```python
from build123d import *

# Parameters (mm, degrees)
SKETCH1_W           = 14.3764
SKETCH1_H           = 14.478
SKETCH1_R           = 0.889
BOSS_EXTRUDE1_DEPTH = 1.8415
SKETCH2_R           = 0.92075
BOSS_EXTRUDE2_DEPTH = 1.27
SKETCH2_4_R         = 0.92075
BOSS_EXTRUDE3_DEPTH = 3.175
FILLET1_R           = 0.762
FILLET2_R           = 0.254


with BuildPart() as part:
    # Sketch1 → Boss-Extrude1 (new body)
    with BuildSketch(Plane(origin=(0, 0, 0), x_dir=(1, 0, 0), z_dir=(0, 1, 0))):
        Rectangle(SKETCH1_W, SKETCH1_H)
        with Locations((-2.6162, 5.1435)):
            Circle(SKETCH1_R, mode=Mode.SUBTRACT)
        with Locations((-2.6162, -5.1435)):
            Circle(SKETCH1_R, mode=Mode.SUBTRACT)
    extrude(amount=BOSS_EXTRUDE1_DEPTH)

    # Sketch2 → Boss-Extrude2 (add, symmetric)
    with BuildSketch(Plane.XY):
        with BuildLine():
            Line((0.848172569, 7.926885609), (-4.6482, 1.8415))
            Line((-4.6482, 1.8415), (5.93687295, 1.8415))
            Line((5.93687295, 1.8415), (5.93687295, 5.969))
            ThreePointArc((5.93687295, 5.969), (4.064774324, 8.695178077), (0.848172569, 7.926885609))
        make_face()
        with Locations((3.01587295, 5.969)):
            Circle(SKETCH2_R, mode=Mode.SUBTRACT)
    extrude(amount=BOSS_EXTRUDE2_DEPTH, both=True)

    # Sketch2<4> → Boss-Extrude3 (add, symmetric)
    with BuildSketch(Plane.XY):
        with Locations((3.01587295, 5.969)):
            Circle(SKETCH2_4_R)
    extrude(amount=BOSS_EXTRUDE3_DEPTH, both=True)

    # Fillet1
    fillet1_edges = [part.edges().sort_by_distance(p)[0] for p in [
        (7.1882, 1.8415, 0),
        (0, 1.8415, -7.239),
        (-4.6482, 1.8415, 0),
        (-7.1882, 1.8415, 0),
        (-7.1882, 0.92075, -7.239),
        (7.1882, 0.92075, -7.239),
        (7.1882, 0.92075, 7.239),
        (-7.1882, 0.92075, 7.239),
        (0, 1.8415, 7.239),
    ]]
    fillet(fillet1_edges, radius=FILLET1_R)

    # Fillet2
    fillet2_edges = [part.edges().sort_by_distance(p)[0] for p in [
        (2.09512295, 5.969, -3.175),
        (2.09512295, 5.969, 3.175),
    ]]
    fillet(fillet2_edges, radius=FILLET2_R)


solid = part.part
```
Can you work these out from the model? Positions are in its coordinate system, mm. A direction names the side the tool comes from. Coordinates: 2 decimals unless noted, no trailing zeros. Loops run counter-clockwise (first coordinate to the right, second up) from the corner with the lowest first, then second, coordinate; pieces in that order, holes last. Notation, with made-up numbers: (-2.75, 11.5) - (42.25, 11.5) arc R19 ccw to (42.25, 31.5) - close; hole circle Ø1 at (-17, 30.25). An arc over 180 degrees is marked (long way). Answer as CSV lines item,"result". Start each with the question number.
1) Thinking about a two-plate mould opening in Z: for faces 1 (the cylindrical face through (2.82, 5.07, 2.11)), 2 (the flat face through (2, 5, -1.27)), 3 (the cylindrical face through (-2.138, 0.908, -5.893)), which applies, pulls with the +Z half, pulls with the -Z half, needs draft (parallel to the pull), parting line crosses it, or undercut?
2) I need wall thicknesses on line 1 (Y direction, x = 3, z = 2); line 2 (Z direction, x = 3.75, y = 3.75); line 3 (Y direction, x = 5.25, z = -1.5). Which ranges of each line are inside material? Lowest first, please. Write a range as from..to.
3) Suppose I cut it at A-A (z = -1.5). Please give me the cut outline in (x, y).
4) For pin 1 (0.8 mm diameter, centred on y = 5, z = 0, fed in from +X); pin 2 (2.5 mm diameter, centred on x = -2.62, z = 5.14, fed in from +Y); pin 3 (3 mm diameter, centred on x = -2.5, y = 3, fed in from -Z), each with a flat end and sliding along its axis, tell me the tip position at first contact or that it passes through.
5) Which directions (+Z, -Z, +X, -X, +Y, -Y) give clear straight access to the entire face, cutting with the end or side of a thin tool? Please do faces 4 (the flat face through (5.937, 4, 0)), 5 (the flat face through (3, 6, 3.175)), 6 (the cylindrical face through (2.82, 5.07, -2.08)).
6) Suppose I cut it at B-B (x = 4.75). Please give me the cut outline in (y, z).
7) Suppose I cut it at C-C (z = 4). Please give me the cut outline in (x, y), plus the area to 3 significant figures.
8) Suppose I cut it at D-D (y = 4.25). Please give me the cut outline in (x, z), plus the area to 3 significant figures.
Check result:
1,face 1,"needs draft"
1,face 2,"pulls with the -Z half"
1,face 3,"undercut"
2,line 1,"y = 0..1.84, 5.05..6.89"
2,line 2,"z = -1.27..1.27"
2,line 3,"y = 0..1.84"
3,outline,"(-7.19, 0) - (7.19, 0) - (7.19, 1.08) arc R0.76 ccw to (6.43, 1.84) - (-6.43, 1.84) arc R0.76 ccw to (-7.19, 1.08) - close; circle Ø1.84 at (3.02, 5.97)"
4,pin 1,"stops at x = 5.94"
4,pin 2,"stops at y = 1.84"
4,pin 3,"stops at z = -7.11"
5,face 4,"+Z, -Z, +X, +Y"
5,face 5,"+Z, +X, -X, +Y"
5,face 6,"-Z"
6,outline,"(0, -7.24) - (1.08, -7.24) arc R0.76 ccw to (1.84, -6.48) - (1.84, -1.27) - (8.32, -1.27) - (8.32, 1.27) - (1.84, 1.27) - (1.84, 6.48) arc R0.76 ccw to (1.08, 7.24) - (0, 7.24) - close"
7,outline,"(-7.19, 0) - (7.19, 0) - (7.19, 1.08) arc R0.76 ccw to (6.43, 1.84) - (-6.43, 1.84) arc R0.76 ccw to (-7.19, 1.08) - close"
7,area,"26.2 mm²"
8,outline,"(-2.47, -1.27) - (5.94, -1.27) - (5.94, 1.27) - (-2.47, 1.27) - close"
8,area,"21.4 mm²"
